Build history of the part. All positions in model axes, mm. A direction names the side the tool comes from. Coordinates: 2 decimals unless noted, no trailing zeros. Write each loop counter-clockwise with the first axis right and the second up, starting at its lowest first coordinate (ties: lowest second). Pieces come first, ordered by that corner, then holes.
```python
from build123d import *

# Parameters (mm, degrees)
BOSS_EXTRUDE1_DEPTH = 25
CUT_EXTRUDE2_DEPTH  = 26
BOSS_EXTRUDE2_DEPTH = 0.4


with BuildPart() as part:
    # Sketch1 → Boss-Extrude1 (new body)
    with BuildSketch(Plane(origin=(0, 0, 0), x_dir=(1, 0, 0), z_dir=(0, 1, 0))):
        with BuildLine():
            ThreePointArc((1.451818925, -34.068556857), (1.641248992, -34.346908706), (1.964225605, -34.442038138))
            ThreePointArc((1.964225605, -34.442038138), (26.591847487, -21.978073076), (34.198225299, 4.555174015))
            ThreePointArc((34.198225299, 4.555174015), (23.590291339, 25.176355888), (2.324135821, 34.423627607))
            ThreePointArc((2.324135821, 34.423627607), (1.751838249, 34.289058819), (1.354061739, 33.856153382))
            ThreePointArc((1.354061739, 33.856153382), (0, 33.001534515), (-1.354061739, 33.856153382))
            ThreePointArc((-1.354061739, 33.856153382), (-1.751838249, 34.289058819), (-2.324135821, 34.423627607))
            ThreePointArc((-2.324135821, 34.423627607), (-23.590291339, 25.176355888), (-34.198225299, 4.555174015))
            ThreePointArc((-34.198225299, 4.555174015), (-26.591847487, -21.978073076), (-1.964225605, -34.442038138))
            ThreePointArc((-1.964225605, -34.442038138), (-1.641248992, -34.346908706), (-1.451818925, -34.068556857))
            ThreePointArc((-1.451818925, -34.068556857), (0, -32.945679925), (1.451818925, -34.068556857))
        make_face()
        with BuildLine():
            Line((-2.417, 3.787737139), (0, 3.787737139))
            Line((0, 3.787737139), (2.417, 3.787737139))
            ThreePointArc((2.417, 3.787737139), (0, -4.489512172), (-2.417, 3.787737139))
        make_face(mode=Mode.SUBTRACT)
    extrude(amount=BOSS_EXTRUDE1_DEPTH)

    # Sketch2 → Cut-Extrude2 (cut, through all)
    with BuildSketch(Plane(origin=(0, 0, 0), x_dir=(1, 0, 0), z_dir=(0, 1, 0))):
        with BuildLine():
            ThreePointArc((-30.913793103, -2.310280493), (-21.920310217, -21.920310217), (-2.310280493, -30.913793103))
            ThreePointArc((-2.310280493, -30.913793103), (-1.447519283, -30.787674087), (-0.720410046, -30.306451613))
            ThreePointArc((-0.720410046, -30.306451613), (0, -30), (0.720410046, -30.306451613))
            ThreePointArc((0.720410046, -30.306451613), (1.447519283, -30.787674087), (2.310280493, -30.913793103))
            ThreePointArc((2.310280493, -30.913793103), (21.920310217, -21.920310217), (30.913793103, -2.310280493))
            ThreePointArc((30.913793103, -2.310280493), (30.787674087, -1.447519283), (30.306451613, -0.720410046))
            ThreePointArc((30.306451613, -0.720410046), (30, 0), (30.306451613, 0.720410046))
            ThreePointArc((30.306451613, 0.720410046), (30.787674087, 1.447519283), (30.913793103, 2.310280493))
            ThreePointArc((30.913793103, 2.310280493), (21.920310217, 21.920310217), (2.310280493, 30.913793103))
            ThreePointArc((2.310280493, 30.913793103), (1.447519283, 30.787674087), (0.720410046, 30.306451613))
            ThreePointArc((0.720410046, 30.306451613), (0, 30), (-0.720410046, 30.306451613))
            ThreePointArc((-0.720410046, 30.306451613), (-1.447519283, 30.787674087), (-2.310280493, 30.913793103))
            ThreePointArc((-2.310280493, 30.913793103), (-21.920310217, 21.920310217), (-30.913793103, 2.310280493))
            ThreePointArc((-30.913793103, 2.310280493), (-30.787674087, 1.447519283), (-30.306451613, 0.720410046))
            ThreePointArc((-30.306451613, 0.720410046), (-30, 0), (-30.306451613, -0.720410046))
            ThreePointArc((-30.306451613, -0.720410046), (-30.787674087, -1.447519283), (-30.913793103, -2.310280493))
        make_face()
    extrude(amount=CUT_EXTRUDE2_DEPTH, mode=Mode.SUBTRACT)

    # Sketch2<2> → Boss-Extrude2 (add)
    with BuildSketch(Plane(origin=(0, 0, 0), x_dir=(1, 0, 0), z_dir=(0, 1, 0))):
        with BuildLine():
            ThreePointArc((-30.913793103, -2.310280493), (-21.920310217, -21.920310217), (-2.310280493, -30.913793103))
            ThreePointArc((-2.310280493, -30.913793103), (-1.447519283, -30.787674087), (-0.720410046, -30.306451613))
            ThreePointArc((-0.720410046, -30.306451613), (0, -30), (0.720410046, -30.306451613))
            ThreePointArc((0.720410046, -30.306451613), (1.447519283, -30.787674087), (2.310280493, -30.913793103))
            ThreePointArc((2.310280493, -30.913793103), (21.920310217, -21.920310217), (30.913793103, -2.310280493))
            ThreePointArc((30.913793103, -2.310280493), (30.787674087, -1.447519283), (30.306451613, -0.720410046))
            ThreePointArc((30.306451613, -0.720410046), (30, 0), (30.306451613, 0.720410046))
            ThreePointArc((30.306451613, 0.720410046), (30.787674087, 1.447519283), (30.913793103, 2.310280493))
            ThreePointArc((30.913793103, 2.310280493), (21.920310217, 21.920310217), (2.310280493, 30.913793103))
            ThreePointArc((2.310280493, 30.913793103), (1.447519283, 30.787674087), (0.720410046, 30.306451613))
            ThreePointArc((0.720410046, 30.306451613), (0, 30), (-0.720410046, 30.306451613))
            ThreePointArc((-0.720410046, 30.306451613), (-1.447519283, 30.787674087), (-2.310280493, 30.913793103))
            ThreePointArc((-2.310280493, 30.913793103), (-21.920310217, 21.920310217), (-30.913793103, 2.310280493))
            ThreePointArc((-30.913793103, 2.310280493), (-30.787674087, 1.447519283), (-30.306451613, 0.720410046))
            ThreePointArc((-30.306451613, 0.720410046), (-30, 0), (-30.306451613, -0.720410046))
            ThreePointArc((-30.306451613, -0.720410046), (-30.787674087, -1.447519283), (-30.913793103, -2.310280493))
        make_face()
    extrude(amount=BOSS_EXTRUDE2_DEPTH)


solid = part.part
```
1. Saw through at C-C on x = -22. List the corners of the cut face in (y, z).
Computed values:
outline: (0, -26.58) - (25, -26.58) - (25, -21.84) - (0.4, -21.84) - (0.4, 21.84) - (25, 21.84) - (25, 26.57) - (0, 26.57) - close
2. Saw through at A-A on y = 22.75. List the corners of the cut face in (x, z).
Computed values:
outline: (-2.32, -34.42) arc R1 ccw to (-1.35, -33.86) arc R1.5 cw to (1.35, -33.86) arc R1 ccw to (2.32, -34.42) arc R34.5 ccw to (1.96, 34.44) arc R0.5 ccw to (1.45, 34.07) arc R1.5 cw to (-1.45, 34.07) arc R0.5 ccw to (-1.96, 34.44) arc R34.5 ccw to start; hole (-30.91, -2.31) arc R31 ccw to (-2.31, -30.91) arc R2 ccw to (-0.72, -30.31) arc R1 cw to (0.72, -30.31) arc R2 ccw to (2.31, -30.91) arc R31 ccw to (30.91, -2.31) arc R2 ccw to (30.31, -0.72) arc R1 cw to (30.31, 0.72) arc R2 ccw to (30.91, 2.31) arc R31 ccw to (2.31, 30.91) arc R2 ccw to (0.72, 30.31) arc R1 cw to (-0.72, 30.31) arc R2 ccw to (-2.31, 30.91) arc R31 ccw to (-30.91, 2.31) arc R2 ccw to (-30.31, 0.72) arc R1 cw to (-30.31, -0.72) arc R2 ccw to start
3. Mould opens along Z. For faces 1 (the face through (-31, 25, 0)), 2 (the face through (-30.792, 12.528, -1.459)), 3 (the face through (0, 12, -33)) say: +Z half, -Z half, draft (parallel to the pull), parting line (faces both ways), or undercut.
Computed values:
face 1: draft
face 2: undercut
face 3: -Z half
4. Probe line 1 along X through (y, z) = (6.25, -2); line 2 along Y through (x, z) = (-14.5, -27); line 3 along X through (y, z) = (21.25, 7). List the from-to ranges inside material, lowest first.
Computed values:
line 1: x = -34.44 to -30.91, 30.91 to 34.44
line 2: y = 0 to 0.4
line 3: x = -33.78 to -30.2, 30.2 to 33.78
5. Saw through at B-B on z = 17. List the corners of the cut face in (x, y).
Computed values:
outline: (-30.02, 0) - (30.02, 0) - (30.02, 25) - (25.92, 25) - (25.92, 0.4) - (-25.92, 0.4) - (-25.92, 25) - (-30.02, 25) - close
6. Flat gauge pins, fed straight in: pin 1 (2 mm diameter, centred on x = -11.5, z = -9, fed in from +Y); pin 2 (8 mm diameter, centred on x = -26.5, z = -12, fed in from +Y); pin 3 (2 mm diameter, centred on y = 17, z = -12, fed in from -X); pin 4 (5 mm diameter, centred on x = -9.5, y = 21, fed in from -Z). Where does each tip first touch, or does it go through?
Computed values:
pin 1: stops at y = 0.4
pin 2: stops at y = 25
pin 3: stops at x = -32.7
pin 4: stops at z = -33.78
7. 3-axis set-ups, long thin cutter, end or side, ignore diameter. For faces 4 (the face through (1.459, 12.528, -30.792)), 5 (the face through (-0.028, 12.325, 32.946)): which of +Z, -Z, +X, -X, +Y, -Y reach the whole face in a straight line?
Computed values:
face 4: +Y
face 5: +Z, +Y, -Y
